The model under review builds one solid part; all positions refer to its coordinate system, in mm. A direction names the side the tool comes from. Give positions to 0.01 mm unless a question says otherwise; leave off trailing zeros. Order: outer loops, then holes, each group sorted by start corner. A loop starts at its lowest first (then second) coordinate and runs counter-clockwise, first axis right, second up. Notation, with made-up numbers: (6, -30) -> (33, -30) arc R32 cw to (33, 9) -> close; hole circle Ø9 at (-23.75, 15.25). An arc over 180 degrees is marked (long way). Use one line per item in the form item = value.
```python
from build123d import *

# Parameters (mm, degrees)
BOSS_EXTRUDE1_DEPTH      = 19
CUT_EXTRUDE1_DEPTH       = 204.4330356653019
CUT_EXTRUDE1_DEPTH_BACK  = 204.4330356653019
SHELL1_T                 = -4
SHELL1_THICKNESS_2_DEPTH = 5
FILLET2_R                = 2
FILLET3_R                = 2
BOSS_EXTRUDE2_DEPTH      = 1.9999999999999862
CHAMFER1_SIZE            = 1
CHAMFER2_SIZE            = 1
CUT_EXTRUDE2_DEPTH       = 1.6
CUT_EXTRUDE3_DEPTH       = 25.000000000000007


with BuildPart() as part:
    # Sketch1 → Boss-Extrude1 (new body)
    with BuildSketch(Plane(origin=(0, 0, 0), x_dir=(1, 0, 0), z_dir=(0, 1, 0))):
        Polygon((15, 1.84e-15), (-15, -1.84e-15), (-31.99999999999997, -200), (32.00000000000003, -200), align=None)
    extrude(amount=BOSS_EXTRUDE1_DEPTH)

    # Sketch4 → Cut-Extrude1 (cut, two sides: drawn at the far end of the back side and taken through both)
    with BuildSketch(Plane(origin=(0, 0, 0), x_dir=(0, 0, -1), z_dir=(1, 0, 0)).offset(-CUT_EXTRUDE1_DEPTH_BACK)):
        Polygon((-200, 0), (0, 0), (1.59e-15, 2), align=None)
    extrude(amount=CUT_EXTRUDE1_DEPTH + CUT_EXTRUDE1_DEPTH_BACK, mode=Mode.SUBTRACT)

    # Shell1
    shell1_openings = [part.faces().sort_by_distance(p)[0] for p in [
        (0, 0.879432624, 112.056737589),
    ]]
    offset(amount=SHELL1_T, openings=shell1_openings, kind=Kind.INTERSECTION)

    # Shell1 thickness 2 face (on inner face of the shell) → Shell1 thickness 2 (add)
    with BuildSketch(Plane(origin=(0, 15, 113.400681607), x_dir=(0, 0, 1), z_dir=(0, 1, 0))):
        Polygon((-109.400681607, 11.325576006448747), (82.599318393, 27.645576006448778), (82.599318393, -27.645576006448714), (-109.400681607, -11.325576006448745), align=None)
    extrude(amount=-SHELL1_THICKNESS_2_DEPTH)

    # Fillet2
    fillet2_edges = [part.edges().sort_by_distance(p)[0] for p in [
        (23.500000000000014, 0.9999999999999999, 100.00000000000001),
        (19.485576006448763, 1.0000000000000002, 100),
    ]]
    fillet(fillet2_edges, radius=FILLET2_R - 0.0001)  # a hair under: the kernel refuses the full size

    # Fillet3
    fillet3_edges = [part.edges().sort_by_distance(p)[0] for p in [
        (-23.499999999999986, 1, 100),
        (-19.48557600644873, 0.9999999999999998, 100),
    ]]
    fillet(fillet3_edges, radius=FILLET3_R - 0.0001)  # a hair under: the kernel refuses the full size

    # Sketch5 → Boss-Extrude2 (add)
    with BuildSketch(Plane(origin=(0, 19, 0), x_dir=(1, 0, 0), z_dir=(0, 1, 0))):
        Polygon((-15, -1.84e-15), (-15.169255888521393, -1.9912457473105094), (15.169255888521398, -1.9912457473105094), (15, 1.84e-15), align=None)
    extrude(amount=BOSS_EXTRUDE2_DEPTH)

    # Chamfer1
    chamfer1_edges = [part.edges().sort_by_distance(p)[0] for p in [
        (23.58462794426071, 19, 100.99562287365525),
        (-23.58462794426068, 19, 100.99562287365526),
    ]]
    chamfer(chamfer1_edges, length=CHAMFER1_SIZE)

    # Chamfer2
    chamfer2_edges = [part.edges().sort_by_distance(p)[0] for p in [
        (-15.084627944260696, 20.999999999999986, 0.9956228736552557),
        (15.0846279442607, 20.999999999999986, 0.9956228736552538),
    ]]
    chamfer(chamfer2_edges, length=CHAMFER2_SIZE)

    # Sketch6 → Cut-Extrude2 (cut)
    with BuildSketch(Plane(origin=(0, 19, 0), x_dir=(1, 0, 0), z_dir=(0, 1, 0))):
        Polygon((-14.165649890133558, -1.9912457473105094), (14.16564989013358, -1.9912457473105079), (30.825649890133608, -197.99124574731053), (-30.825649890133526, -197.99124574731053), align=None)
    extrude(amount=-CUT_EXTRUDE2_DEPTH, mode=Mode.SUBTRACT)

    # Sketch7 → Cut-Extrude3 (cut)
    with BuildSketch(Plane.XY.offset(200)):
        Polygon((-31.99999999999997, 9.99920305283565), (32.00000000000003, 9.999203052835664), (32.00000000000003, 0), (-31.99999999999997, 0), align=None)
    extrude(amount=-CUT_EXTRUDE3_DEPTH, mode=Mode.SUBTRACT)


solid = part.part
```
1. The part is to be moulded in two halves that separate along X. For faces 1 (the face through (-21.73, 1.71, 86.24)), 2 (the face through (19.067, 1.719, 88.334)), 3 (the face through (0, 14, 200)), say which applies: +X half, -X half, draft (parallel to the pull), parting line (faces both ways), or undercut.
Values:
face_1 = -X half
face_2 = undercut
face_3 = draft
2. Add section B-B on y = 14.25. Give the boundary of the cut face in (x, z).
Values:
outline = (-32, 200) -> (-15, 0) -> (15, 0) -> (32, 200) -> close
3. For L1, parallel to Y at x = 12, z = 86; L2, parallel to X at y = 5.75, z = 123 (3 decimals); L3, parallel to X at y = 7.5, z = 133 (3 decimals), list the stretches that pass through material, from the lowest coordinate up.
Values:
L1 = 10 to 17.4
L2 = -25.455 to -21.441, 21.441 to 25.455
L3 = -26.305 to -22.291, 22.291 to 26.305
4. For pin 1 Ø2 at (x, y) = (5, 8) entering from +Z; pin 2 Ø8 at (x, z) = (21, 107) entering from -Y; pin 3 Ø2 at (x, y) = (-28, 3.5) entering from +Z, all flat-tipped, find the tip position at first contact; note any pin that passes through.
Values:
pin_1 = 4
pin_2 = 0.89
pin_3 = 175
5. Tool access review of faces 4 (the face through (-22.61, 18.21, 101.36)), 5 (the face through (-19.37, 6.07, 98.66)), 6 (the face through (0, 9.999, 199)): name each direction out of +Z, -Z, +X, -X, +Y, -Y from which nothing blocks a thin tool from reaching the whole face with its end or side.
Values:
face_4 = +Y
face_5 = +Z, -Y
face_6 = +Z, +X, -X, -Y
